```python
from build123d import *

# Parameters (mm, degrees)
SKETCH_1_R                   = 45
SKETCH_1_R_2                 = 19.01
EXTRUDE_1_DEPTH              = 10
HOLE_WIZARD_M4_1_D           = 3.3
HOLE_WIZARD_M4_1_DEPTH       = 10.1
HOLE_WIZARD_M4_1_CBORE_D     = 4
HOLE_WIZARD_M4_1_CBORE_DEPTH = 8
HOLE_WIZARD_M4_1_TIP         = 0.991420021
SKETCH_4_R                   = 4.2
CUT_EXTRUDE_1_DEPTH          = 10


with BuildPart() as part:
    # 草图1 → 拉伸1 (new body)
    with BuildSketch(Plane.XY):
        Circle(SKETCH_1_R)
        Circle(SKETCH_1_R_2, mode=Mode.SUBTRACT)
    extrude(amount=EXTRUDE_1_DEPTH)

    # M4 螺纹孔1
    with Locations(Plane(origin=(-23.5, 23.5, 10), x_dir=(1, 0, 0), z_dir=(0, 0, 1))):
        with Locations((0, 0), (47, 0), (47, -47), (0, -47)):
            CounterBoreHole(HOLE_WIZARD_M4_1_D / 2, HOLE_WIZARD_M4_1_CBORE_D / 2, HOLE_WIZARD_M4_1_CBORE_DEPTH, depth=HOLE_WIZARD_M4_1_DEPTH)
            with Locations((0, 0, -(HOLE_WIZARD_M4_1_DEPTH + HOLE_WIZARD_M4_1_TIP / 2))):  # 118° drill point
                Cone(0, HOLE_WIZARD_M4_1_D / 2, HOLE_WIZARD_M4_1_TIP, mode=Mode.SUBTRACT)

    # 草图4 → 切除-拉伸1 (cut)
    with BuildSketch(Plane.XY.offset(10)):
        with Locations((0, 35)):
            Circle(SKETCH_4_R)
        with Locations((-35, 0)):
            Circle(SKETCH_4_R)
        with Locations((0, -35)):
            Circle(SKETCH_4_R)
        with Locations((35, 0)):
            Circle(SKETCH_4_R)
    extrude(amount=-CUT_EXTRUDE_1_DEPTH, mode=Mode.SUBTRACT)


solid = part.part
```
Part model, mm, in its own coordinate system. A direction names the side the tool comes from. Round coordinates to 2 decimals unless told otherwise and drop trailing zeros. Write each loop counter-clockwise with the first axis right and the second up, starting at its lowest first coordinate (ties: lowest second). Pieces come first, ordered by that corner, then holes. Notation, with made-up numbers: (85.5, 20) -> (113.5, 20) arc R8 ccw to (113.5, 26) -> close; hole circle Ø8 at (36, -7). An arc over 180 degrees is marked (long way). Return JSON: item names as keys, results as strings. Group by question number.
Q1. Saw through at B-B on y = 0. Write the cut outline in (x, z).
Q2. Probe L1, parallel to Y at x = 0, z = 4; L2, parallel to Y at x = -23.5, z = 0.5; L3, parallel to Y at x = -5, z = 2.5. List the from-to ranges inside material, lowest first. Write a range as [from, to].
Q3. Saw through at D-D on x = -23.5. Write the cut outline in (y, z).
Q4. Which spindle directions (+Z, -Z, +X, -X, +Y, -Y) get a long thin tool onto all of the face, cutting with end or side? Do faces 4 (the cylindrical face through (24.716, -22.385, 0.986)), 5 (the cylindrical face through (21.502, -23.412, 6.056)). Say none if no direction does.
Q5. Pin check, flat tips, straight feed: pin 1 (1 mm diameter, centred on y = -17.5, z = 7.5, fed in from +X); pin 2 (2 mm diameter, centred on x = 23.5, y = -23.5, fed in from -Z); pin 3 (2 mm diameter, centred on x = 23, y = -23, fed in from +Z). Stop position of each tip, or through.
Q6. Mould opens along Y. For faces 1 (the cylindrical face through (-30.994, 1.262, 5.07)), 2 (the cylindrical face through (20.765, -39.923, 4.93)), 3 (the flat face through (19.4, 0.6, 0)) say: pulls with the +Y half, pulls with the -Y half, needs draft (parallel to the pull), parting line crosses it, or undercut.
Q7. Saw through at A-A on z = 6.75. State how many separate pieces and enclosed holes the cut face has, plus the area to 3 significant figures.
Answer:
{
 "1": {"outline": "(-45, 0) -> (-39.2, 0) -> (-39.2, 10) -> (-45, 10) -> close; (-30.8, 0) -> (-19.01, 0) -> (-19.01, 10) -> (-30.8, 10) -> close; (19.01, 0) -> (30.8, 0) -> (30.8, 10) -> (19.01, 10) -> close; (39.2, 0) -> (45, 0) -> (45, 10) -> (39.2, 10) -> close"},
 "2": {"L1": "[-45, -39.2], [-30.8, -19.01], [19.01, 30.8], [39.2, 45]", "L2": "[-38.38, -25.15], [-21.85, 21.85], [25.15, 38.38]", "L3": "[-44.72, -18.34], [18.34, 44.72]"},
 "3": {"outline": "(-38.38, 0) -> (-25.15, 0) -> (-25.15, 2) -> (-25.5, 2) -> (-25.5, 10) -> (-38.38, 10) -> close; (-21.85, 0) -> (21.85, 0) -> (21.85, 2) -> (21.5, 2) -> (21.5, 10) -> (-21.5, 10) -> (-21.5, 2) -> (-21.85, 2) -> close; (25.15, 0) -> (38.38, 0) -> (38.38, 10) -> (25.5, 10) -> (25.5, 2) -> (25.15, 2) -> close"},
 "4": {"face 4": "+Z, -Z", "face 5": "+Z"},
 "5": {"pin 1": "x = 41.67", "pin 2": "through", "pin 3": "z = 2"},
 "6": {"face 1": "undercut", "face 2": "parting line crosses it", "face 3": "needs draft"},
 "7": {"separate pieces": "1", "enclosed holes": "9", "area": "4,950 mm2"}
}
